Geometry: final body of the model. Coordinates: model frame, mm. A direction names the side the tool comes from. Round coordinates to 2 decimals unless told otherwise and drop trailing zeros. Write each loop counter-clockwise with the first axis right and the second up, starting at its lowest first coordinate (ties: lowest second). Pieces come first, ordered by that corner, then holes. Notation, with made-up numbers: (4.25, 21.25) -> (62.25, 21.25) arc R28 ccw to (62.25, 54.25) -> close; hole circle Ø8 at (-39, -37.75). An arc over 180 degrees is marked (long way). One line per item, written item: value. Start each with the question number.
from build123d import *

# Parameters (mm, degrees)
SKETCH1_W           = 19.05
SKETCH1_H           = 19.05
SKETCH1_W_2         = 15.875
SKETCH1_H_2         = 15.875
EXTRUDE_THIN1_DEPTH = 127
SKETCH2_W           = 19.05
SKETCH2_H           = 19.05
CUT_EXTRUDE1_DEPTH  = 17.4625
SKETCH3_W           = 19.05
SKETCH3_H           = 19.05
CUT_EXTRUDE2_DEPTH  = 17.4625


with BuildPart() as part:
    # Sketch1 → Extrude-Thin1 (new body)
    with BuildSketch(Plane(origin=(0, 0, 0), x_dir=(1, 0, 0), z_dir=(0, 1, 0))):
        with Locations((9.525, 9.525)):
            Rectangle(SKETCH1_W, SKETCH1_H)
        with Locations((9.525, 9.525)):
            Rectangle(SKETCH1_W_2, SKETCH1_H_2, mode=Mode.SUBTRACT)
    extrude(amount=EXTRUDE_THIN1_DEPTH)

    # Sketch2 → Cut-Extrude1 (cut)
    with BuildSketch(Plane.ZY):
        with Locations((-9.525, 9.525)):
            Rectangle(SKETCH2_W, SKETCH2_H)
    extrude(amount=-CUT_EXTRUDE1_DEPTH, mode=Mode.SUBTRACT)

    # Sketch3 → Cut-Extrude2 (cut)
    with BuildSketch(Plane.ZY):
        with Locations((-9.525, 117.475)):
            Rectangle(SKETCH3_W, SKETCH3_H)
    extrude(amount=-CUT_EXTRUDE2_DEPTH, mode=Mode.SUBTRACT)


solid = part.part
(1) Pull-direction query (Z, two-part tool) for faces 1 (the face through (17.462, 64, -10)), 2 (the face through (9, 63, -19.05)), 3 (the face through (9, 63, 0)); classes: pulls with the +Z half, pulls with the -Z half, needs draft (parallel to the pull), parting line crosses it, or undercut.
(2) Section query D-D (y = 117). Output: boundary loops of the cut face in (x, z).
(3) Set-up query: faces 4 (the face through (0, 63, -9)), 5 (the face through (1, 19.05, -10)), 6 (the face through (19.05, 63, -9)), 7 (the face through (9, 63, -1.588)), 8 (the face through (1, 107.95, -10)). Return all of +Z, -Z, +X, -X, +Y, -Y with unobstructed straight access to the full face (end or side cutting, diameter ignored); none if empty.
(4) Section query A-A (z = -15.75). Output: boundary loops of the cut face in (x, y).
(5) Section query B-B (x = 10). Output: boundary loops of the cut face in (y, z).
(6) Section query C-C (y = 32.5). Output: boundary loops of the cut face in (x, z).
(7) Pin query (flat end, axial travel): pin 1 (8.5 mm diameter, centred on x = 13, z = -11, fed in from -Y); pin 2 (2 mm diameter, centred on x = 2.5, z = -15, fed in from -Y). Return the tip coordinate at first contact, or that it passes through.
(8) Line query: probe 1 along Z at (x, y) = (8.25, 69.5); probe 2 along X at (y, z) = (58, -9.25); probe 3 along Y at (x, z) = (10, -1.5). Output: solid intervals per line, ascending.
Results list:
1. face 1: undercut
1. face 2: pulls with the -Z half
1. face 3: pulls with the +Z half
2. outline: (17.46, -19.05) -> (19.05, -19.05) -> (19.05, 0) -> (17.46, 0) -> close
3. face 4: +Z, -Z, -X, +Y, -Y
3. face 5: +Z, -Z, -X, -Y
3. face 6: +Z, -Z, +X, +Y, -Y
3. face 7: +Y, -Y
3. face 8: +Z, -Z, -X, +Y
4. outline: (0, 19.05) -> (1.59, 19.05) -> (1.59, 107.95) -> (0, 107.95) -> close; (17.46, 0) -> (19.05, 0) -> (19.05, 127) -> (17.46, 127) -> close
5. outline: (19.05, -19.05) -> (107.95, -19.05) -> (107.95, -17.46) -> (19.05, -17.46) -> close; (19.05, -1.59) -> (107.95, -1.59) -> (107.95, 0) -> (19.05, 0) -> close
6. outline: (0, -19.05) -> (19.05, -19.05) -> (19.05, 0) -> (0, 0) -> close; hole (1.59, -17.46) -> (17.46, -17.46) -> (17.46, -1.59) -> (1.59, -1.59) -> close
7. pin 1: passes through
7. pin 2: stops at y = 19.05
8. probe 1: z = -19.05 to -17.46, -1.59 to 0
8. probe 2: x = 0 to 1.59, 17.46 to 19.05
8. probe 3: y = 19.05 to 107.95
